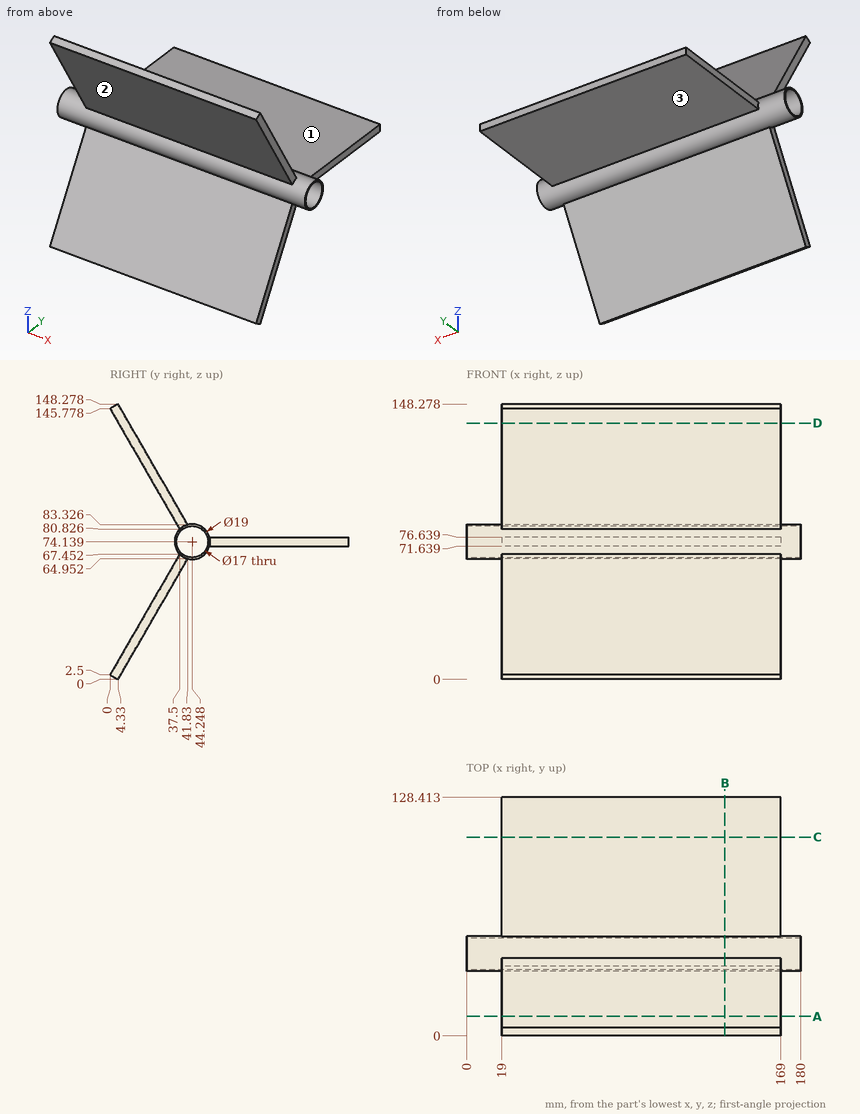
Design review of the part shown in the three views and the two pictorial views. Dimensions are in mm from the part's minimum x, y and z. Give positions to 0.01 mm unless a question says otherwise; leave off trailing zeros. Write each loop counter-clockwise with the first axis right and the second up, starting at its lowest first coordinate (ties: lowest second). Pieces come first, ordered by that corner, then holes.
Item 1: Take a section at B-B (x = 139). Give the boundary of the cut face in (y, z).
Item 2: Insertion check: P1, Ø22.5, axis at x = 123, y = 78.5, coming from the +Z side; P2, Ø5, axis at x = 35, y = 42.5, coming from the -Z side; P3, Ø1.5, axis at y = 101.5, z = 74, coming from the +X side. Each pin has a flat end and moves straight along its axis. Give the tip position at first contact, or say it passes through.
Item 3: Take a section at D-D (z = 138). Give the boundary of the cut face in (x, y) (1 decimal), and give its area (3 significant figures).
Item 4: Take a section at C-C (y = 107). Give the boundary of the cut face in (x, z).
Item 5: The part is to be moulded in two halves that separate along Z. For the marked faces 1, 2 and 3, say which applies: +Z half, -Z half, draft (parallel to the pull), parting line (faces both ways), or undercut.
Item 6: Take a section at A-A (y = 10.5). Give the boundary of the cut face in (x, z), and give its area (3 significant figures).
Item 7: Wall thickness on probe 1 along Z at (x, y) = (142, 48) (1 decimal); probe 2 along X at (y, z) = (24, 44); probe 3 along Y at (x, z) = (82.5, 67) (1 decimal): over which ranges is each line inside the solid? List them lowest first.
Established:
1. outline: (0, 2.5) - (4.33, 0) - (41.83, 64.95) arc R9.5 ccw to (53.41, 71.64) - (128.41, 71.64) - (128.41, 76.64) - (53.41, 76.64) arc R9.5 ccw to (41.83, 83.33) - (4.33, 148.28) - (0, 145.78) - (37.5, 80.83) arc R9.5 ccw to (37.5, 67.45) - close; hole circle Ø17 at (44.25, 74.14)
2. P1: stops at z = 76.64
2. P2: stops at z = 61.78
2. P3: stops at x = 169
3. outline: (19, 4.5) - (169, 4.5) - (169, 10.3) - (19, 10.3) - close
3. area: 866 mm2
4. outline: (19, 71.64) - (169, 71.64) - (169, 76.64) - (19, 76.64) - close
5. face 1: +Z half
5. face 2: undercut
5. face 3: -Z half
6. outline: (19, 10.69) - (169, 10.69) - (169, 20.69) - (19, 20.69) - close; (19, 127.59) - (169, 127.59) - (169, 137.59) - (19, 137.59) - close
6. area: 3,000 mm2
7. probe 1: z = 65.4 to 66.5, 81.8 to 82.9
7. probe 2: x = 19 to 169
7. probe 3: y = 37.2 to 39.6, 48.9 to 50.5
